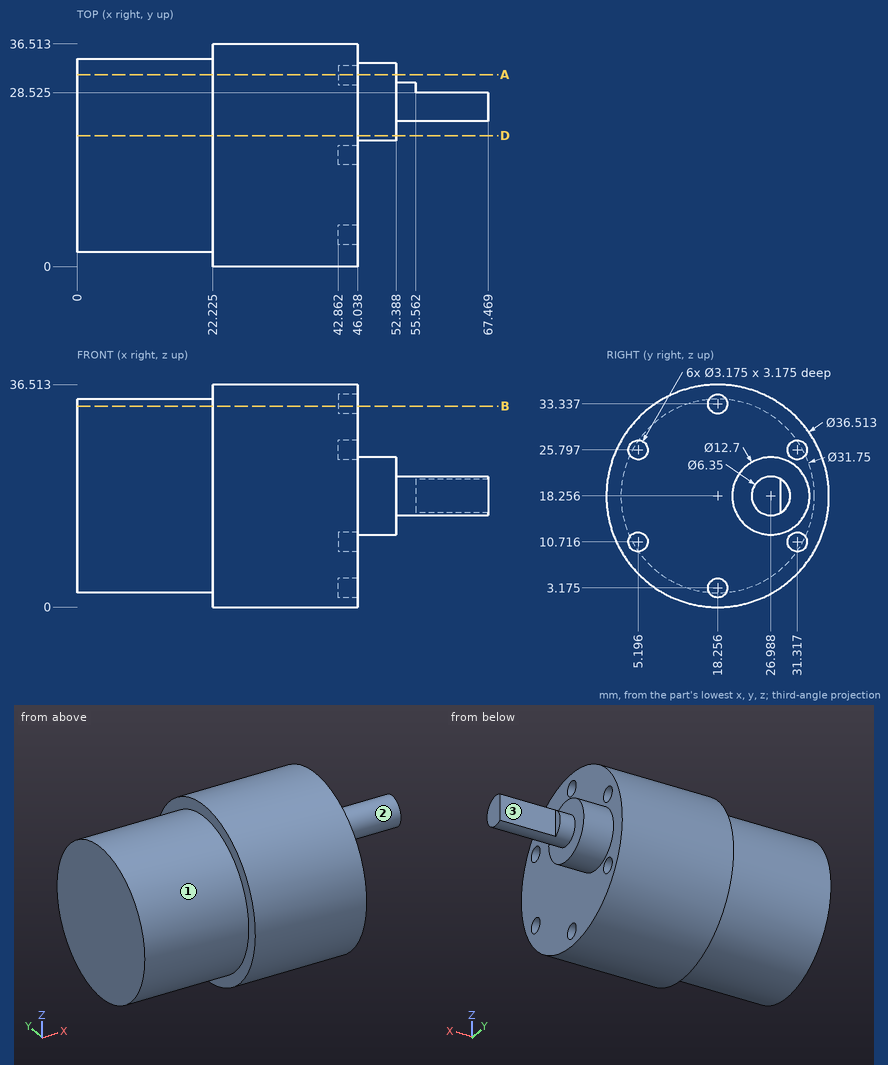
For this review, use the dimensioned drawing (mm, ordinates from the lowest corner) and the shaded views. A direction names the side the tool comes from. Give positions to 0.01 mm unless a question says otherwise; leave off trailing zeros. Loops run counter-clockwise (first coordinate to the right, second up) from the corner with the lowest first, then second, coordinate; pieces in that order, holes last. Notation, with made-up numbers: (-19.5, 20.25) -> (-1.5, 20.25) arc R6 ccw to (-1.5, 30.25) -> close; hole circle Ø8 at (89, 87.25). An arc over 180 degrees is marked (long way). One line per question, with ' | ' between items. Start each with the question number.
(1) We need section B-B (z = 33). State the section outline as (x, y) points (1 decimal).
(2) Insertion check: P1, Ø3, axis at y = 5.2, z = 25.8, coming from the +X side; P2, Ø12, axis at x = 55.5, y = 20, coming from the -Z side (1 decimal); P3, Ø0.8, axis at y = 29, z = 17.5, coming from the +X side. Each pin has a flat end and moves straight along its axis. Give the tip position at first contact, or say it passes through.
(3) We need section D-D (y = 21.5). State the section outline as (x, z) points (1 decimal), and give its area (3 significant figures).
(4) For line 1 (Z direction, x = 45, y = 5.5) (1 decimal); line 2 (X direction, y = 28, z = 9); line 3 (X direction, y = 32, z = 20), list the stretches that pass through material, from the lowest coordinate up.
(5) For the marked faces 1, 2 and 3, list the 3-axis set-ups (+Z, -Z, +X, -X, +Y, -Y) from which the entire face can be reached by the end or side of a thin tool; tool diameter is ignored.
(6) We need section A-A (y = 31.5). State the section outline as (x, z) points (1 decimal).
The answers:
1) outline: (0, 12.4) -> (22.2, 12.4) -> (22.2, 7.5) -> (46, 7.5) -> (46, 16.7) -> (42.9, 16.7) -> (42.9, 19.8) -> (46, 19.8) -> (46, 29) -> (22.2, 29) -> (22.2, 24.1) -> (0, 24.1) -> close
2) P1: stops at x = 42.86 | P2: stops at z = 12.2 | P3: stops at x = 55.56
3) outline: (0, 2.7) -> (22.2, 2.7) -> (22.2, 0.3) -> (46, 0.3) -> (46, 15.1) -> (52.4, 15.1) -> (52.4, 21.5) -> (46, 21.5) -> (46, 36.2) -> (22.2, 36.2) -> (22.2, 33.8) -> (0, 33.8) -> close | area: 1,590 mm^2
4) line 1: z = 5.2 to 9.2, 12.3 to 24.2, 27.4 to 31.3 | line 2: x = 0 to 46.04 | line 3: x = 0 to 52.39
5) face 1: -X | face 2: +X | face 3: +Z, -Z, +X, +Y
6) outline: (0, 9.5) -> (22.2, 9.5) -> (22.2, 5.7) -> (46, 5.7) -> (46, 9.1) -> (42.9, 9.1) -> (42.9, 12.3) -> (46, 12.3) -> (46, 13.8) -> (52.4, 13.8) -> (52.4, 22.7) -> (46, 22.7) -> (46, 24.2) -> (42.9, 24.2) -> (42.9, 27.4) -> (46, 27.4) -> (46, 30.8) -> (22.2, 30.8) -> (22.2, 27) -> (0, 27) -> close
